Input: part model. Units: mm. Frame: model coordinates. A direction names the side the tool comes from. Round coordinates to 2 decimals unless told otherwise and drop trailing zeros. Write each loop counter-clockwise with the first axis right and the second up, starting at its lowest first coordinate (ties: lowest second). Pieces come first, ordered by that corner, then holes. Notation, with made-up numbers: (34.25, 76) - (83.25, 76) arc R29 ccw to (83.25, 109) - close; hole circle Ø4 at (27.25, 52). An arc over 180 degrees is marked (long way). Use one line per item in the form item = value.
```python
from build123d import *

# Parameters (mm, degrees)
SKETCH1_W                      = 38.1
SKETCH1_H                      = 50.8
SKETCH1_W_2                    = 31.75
SKETCH1_H_2                    = 44.45
BOSS_EXTRUDE1_DEPTH            = 152.4
SKETCH2_R                      = 1.89865
CUT_EXTRUDE1_DEPTH             = 35.925
CUT_EXTRUDE1_DEPTH_BACK        = 4.175
CUT_EXTRUDE3_DEPTH             = 3.175
CUT_EXTRUDE4_DEPTH             = 3.175
SKETCH6_R                      = 9.525
SKETCH6_R_2                    = 2.5527
CUT_EXTRUDE5_DEPTH             = 3.175
CUT_EXTRUDE6_DEPTH             = 3.175
F_6_32_TAPPED_HOLE2_D          = 2.7051
F_6_32_TAPPED_HOLE2_DEPTH      = 3.175
CUT_EXTRUDE7_REACH             = 40.1
CUT_EXTRUDE7_DIRECTION_2_DEPTH = 1
FILLET1_R                      = 3.175
FILLET2_R                      = 3.175
BOSS_EXTRUDE2_DEPTH            = 3.175
CUT_EXTRUDE8_REACH             = 40.1
FILLET3_R                      = 3.175
FILLET4_R                      = 3.175
FILLET5_R                      = 6.35
FILLET6_R                      = 6.35
BOSS_EXTRUDE3_DEPTH            = 3.175
CUT_EXTRUDE9_REACH             = 40.1
BOSS_EXTRUDE4_DEPTH            = 3.175
FILLET7_R                      = 3.175
FILLET8_R                      = 3.175
FILLET9_R                      = 3.175
FILLET10_R                     = 3.175
FILLET11_R                     = 6.35
FILLET12_R                     = 6.35


with BuildPart() as part:
    # Sketch1 → Boss-Extrude1 (new body)
    with BuildSketch(Plane(origin=(0, 0, 0), x_dir=(1, 0, 0), z_dir=(0, 1, 0))):
        Rectangle(SKETCH1_W, SKETCH1_H)
        Rectangle(SKETCH1_W_2, SKETCH1_H_2, mode=Mode.SUBTRACT)
    extrude(amount=BOSS_EXTRUDE1_DEPTH)

    # Sketch2 → Cut-Extrude1 (cut, two sides)
    with BuildSketch(Plane.ZY.offset(-15.875)) as cut_extrude1_sk:
        with Locations((-16.645384182, 6.21538)):
            Circle(SKETCH2_R)
        with Locations((10.30030417, 6.18241423)):
            Circle(SKETCH2_R)
    extrude(amount=CUT_EXTRUDE1_DEPTH, mode=Mode.SUBTRACT)
    extrude(cut_extrude1_sk.sketch, amount=-CUT_EXTRUDE1_DEPTH_BACK, mode=Mode.SUBTRACT)

    # Sketch4 → Cut-Extrude3 (cut)
    with BuildSketch(Plane.ZY.offset(19.05)):
        with BuildLine():
            Line((17.4625, 10.16), (-17.4625, 10.16))
            ThreePointArc((-17.4625, 10.16), (-19.70756403, 11.08993597), (-20.6375, 13.335))
            Line((-20.6375, 13.335), (-20.6375, 64.135))
            ThreePointArc((-20.6375, 64.135), (-19.70756403, 66.38006403), (-17.4625, 67.31))
            Line((-17.4625, 67.31), (17.4625, 67.31))
            ThreePointArc((17.4625, 67.31), (19.70756403, 66.38006403), (20.6375, 64.135))
            Line((20.6375, 64.135), (20.6375, 13.335))
            ThreePointArc((20.6375, 13.335), (19.70756403, 11.08993597), (17.4625, 10.16))
        make_face()
    extrude(amount=-CUT_EXTRUDE3_DEPTH, mode=Mode.SUBTRACT)

    # Sketch5 → Cut-Extrude4 (cut)
    with BuildSketch(Plane(origin=(19.05, 0, 0), x_dir=(0, 0, -1), z_dir=(1, 0, 0))):
        with BuildLine():
            Line((17.4625, 67.31), (-17.4625, 67.31))
            ThreePointArc((-17.4625, 67.31), (-19.70756403, 66.38006403), (-20.6375, 64.135))
            Line((-20.6375, 64.135), (-20.6375, 45.085))
            ThreePointArc((-20.6375, 45.085), (-19.70756403, 42.83993597), (-17.4625, 41.91))
            Line((-17.4625, 41.91), (17.4625, 41.91))
            ThreePointArc((17.4625, 41.91), (19.70756403, 42.83993597), (20.6375, 45.085))
            Line((20.6375, 45.085), (20.6375, 64.135))
            ThreePointArc((20.6375, 64.135), (19.70756403, 66.38006403), (17.4625, 67.31))
        make_face()
    extrude(amount=-CUT_EXTRUDE4_DEPTH, mode=Mode.SUBTRACT)

    # Sketch6 → Cut-Extrude5 (cut)
    with BuildSketch(Plane.ZY.offset(-15.875)):
        with Locations((0, 101.6)):
            Circle(SKETCH6_R)
        with Locations((0, 87.63)):
            Circle(SKETCH6_R_2)
        with Locations((-9.878281733, 91.721718267)):
            Circle(SKETCH6_R_2)
        with Locations((-13.97, 101.6)):
            Circle(SKETCH6_R_2)
        with Locations((-9.878281733, 111.478281733)):
            Circle(SKETCH6_R_2)
        with Locations((0, 115.57)):
            Circle(SKETCH6_R_2)
        with Locations((9.878281733, 111.478281733)):
            Circle(SKETCH6_R_2)
        with Locations((13.97, 101.6)):
            Circle(SKETCH6_R_2)
        with Locations((9.878281733, 91.721718267)):
            Circle(SKETCH6_R_2)
    extrude(amount=-CUT_EXTRUDE5_DEPTH, mode=Mode.SUBTRACT)

    # Sketch7 → Cut-Extrude6 (cut)
    with BuildSketch(Plane.ZY.offset(19.05)):
        with BuildLine():
            Line((-14.2875, 77.47), (14.2875, 77.47))
            ThreePointArc((14.2875, 77.47), (18.777628061, 79.329871939), (20.6375, 83.82))
            Line((20.6375, 83.82), (20.6375, 121.92))
            ThreePointArc((20.6375, 121.92), (18.777628061, 126.410128061), (14.2875, 128.27))
            Line((14.2875, 128.27), (-14.2875, 128.27))
            ThreePointArc((-14.2875, 128.27), (-18.777628061, 126.410128061), (-20.6375, 121.92))
            Line((-20.6375, 121.92), (-20.6375, 83.82))
            ThreePointArc((-20.6375, 83.82), (-18.777628061, 79.329871939), (-14.2875, 77.47))
        make_face()
    extrude(amount=-CUT_EXTRUDE6_DEPTH, mode=Mode.SUBTRACT)

    # #6-32 Tapped Hole2
    with Locations(Plane(origin=(5.579615818, 136.6393, -25.4), x_dir=(-1, 0, 0), z_dir=(0, 0, -1))):
        with Locations((0, 0), (11.159231636, 0)):
            Hole(F_6_32_TAPPED_HOLE2_D / 2, depth=F_6_32_TAPPED_HOLE2_DEPTH)

    # Sketch13 → Cut-Extrude7 (cut, up to next)
    with BuildSketch(Plane(origin=(19.05, 0, 0), x_dir=(0, 0, -1), z_dir=(1, 0, 0)), mode=Mode.PRIVATE) as cut_extrude7_sk1:
        Polygon((0, 78.486), (20.6375, 78.486), (20.6375, 64.135), (-20.6375, 64.135), (-20.6375, 78.486), align=None)
    cut_extrude7_tool1 = extrude(cut_extrude7_sk1.sketch, amount=-CUT_EXTRUDE7_REACH, mode=Mode.PRIVATE) & part.part
    add(cut_extrude7_tool1.solids().sort_by_distance((19.05, 71.3105, 0))[0], mode=Mode.SUBTRACT)

    # Sketch13 → Cut-Extrude7 direction 2 (cut)
    with BuildSketch(Plane(origin=(19.05, 0, 0), x_dir=(0, 0, -1), z_dir=(1, 0, 0))):
        Polygon((0, 78.486), (20.6375, 78.486), (20.6375, 64.135), (-20.6375, 64.135), (-20.6375, 78.486), align=None)
    extrude(amount=CUT_EXTRUDE7_DIRECTION_2_DEPTH, mode=Mode.SUBTRACT)

    # Fillet1
    fillet1_edges = [part.edges().sort_by_distance(p)[0] for p in [
        (17.4625, 78.486, -20.6375),
    ]]
    fillet(fillet1_edges, radius=FILLET1_R)

    # Fillet2
    fillet2_edges = [part.edges().sort_by_distance(p)[0] for p in [
        (17.4625, 78.486, 20.6375),
    ]]
    fillet(fillet2_edges, radius=FILLET2_R)

    # Sketch15 → Boss-Extrude2 (add)
    with BuildSketch(Plane.ZY.offset(19.05)):
        Polygon((0, 78.486), (-20.6375, 78.486), (-20.6375, 88.646), (0, 88.646), (20.6375, 88.646), (20.6375, 78.486), align=None)
    extrude(amount=-BOSS_EXTRUDE2_DEPTH)

    # Sketch16 → Cut-Extrude8 (cut, up to next)
    with BuildSketch(Plane.ZY.offset(19.05), mode=Mode.PRIVATE) as cut_extrude8_sk1:
        Polygon((0, 78.486), (20.6375, 78.486), (20.6375, 64.135), (-20.6375, 64.135), (-20.6375, 78.486), align=None)
    cut_extrude8_tool1 = extrude(cut_extrude8_sk1.sketch, amount=-CUT_EXTRUDE8_REACH, mode=Mode.PRIVATE) & part.part
    add(cut_extrude8_tool1.solids().sort_by_distance((-19.05, 71.3105, 0))[0], mode=Mode.SUBTRACT)

    # Fillet3
    fillet3_edges = [part.edges().sort_by_distance(p)[0] for p in [
        (-17.4625, 78.486, 20.6375),
    ]]
    fillet(fillet3_edges, radius=FILLET3_R)

    # Fillet4
    fillet4_edges = [part.edges().sort_by_distance(p)[0] for p in [
        (-17.4625, 78.486, -20.6375),
    ]]
    fillet(fillet4_edges, radius=FILLET4_R)

    # Fillet5
    fillet5_edges = [part.edges().sort_by_distance(p)[0] for p in [
        (-17.4625, 88.646, -20.6375),
    ]]
    fillet(fillet5_edges, radius=FILLET5_R)

    # Fillet6
    fillet6_edges = [part.edges().sort_by_distance(p)[0] for p in [
        (-17.4625, 88.646, 20.6375),
    ]]
    fillet(fillet6_edges, radius=FILLET6_R)

    # Sketch17 → Boss-Extrude3 (add)
    with BuildSketch(Plane.ZY.offset(19.05)):
        Polygon((0, 74.168), (20.6375, 74.168), (20.6375, 84.35471455), (-20.6375, 84.35471455), (-20.6375, 74.168), align=None)
    extrude(amount=-BOSS_EXTRUDE3_DEPTH)

    # Sketch18 → Cut-Extrude9 (cut, up to next)
    with BuildSketch(Plane.ZY.offset(19.05), mode=Mode.PRIVATE) as cut_extrude9_sk1:
        Polygon((0, 84.328), (-20.6375, 84.328), (-20.6375, 94.996), (20.6375, 94.996), (20.6375, 84.328), align=None)
    cut_extrude9_tool1 = extrude(cut_extrude9_sk1.sketch, amount=-CUT_EXTRUDE9_REACH, mode=Mode.PRIVATE) & part.part
    add(cut_extrude9_tool1.solids().sort_by_distance((-19.05, 89.662, 0))[0], mode=Mode.SUBTRACT)

    # Sketch19 → Boss-Extrude4 (add)
    with BuildSketch(Plane(origin=(19.05, 0, 0), x_dir=(0, 0, -1), z_dir=(1, 0, 0))):
        Polygon((0, 74.168), (20.6375, 74.168), (20.6375, 78.486), (-20.6375, 78.486), (-20.6375, 74.168), align=None)
    extrude(amount=-BOSS_EXTRUDE4_DEPTH)

    # Fillet7
    fillet7_edges = [part.edges().sort_by_distance(p)[0] for p in [
        (17.4625, 74.168, -20.6375),
    ]]
    fillet(fillet7_edges, radius=FILLET7_R)

    # Fillet8
    fillet8_edges = [part.edges().sort_by_distance(p)[0] for p in [
        (17.4625, 74.168, 20.6375),
    ]]
    fillet(fillet8_edges, radius=FILLET8_R)

    # Fillet9
    fillet9_edges = [part.edges().sort_by_distance(p)[0] for p in [
        (-17.4625, 74.168, 20.6375),
    ]]
    fillet(fillet9_edges, radius=FILLET9_R)

    # Fillet10
    fillet10_edges = [part.edges().sort_by_distance(p)[0] for p in [
        (-17.4625, 74.168, -20.6375),
    ]]
    fillet(fillet10_edges, radius=FILLET10_R)

    # Fillet11
    fillet11_edges = [part.edges().sort_by_distance(p)[0] for p in [
        (-17.4625, 84.328, -20.6375),
    ]]
    fillet(fillet11_edges, radius=FILLET11_R)

    # Fillet12
    fillet12_edges = [part.edges().sort_by_distance(p)[0] for p in [
        (-17.4625, 84.328, 20.6375),
    ]]
    fillet(fillet12_edges, radius=FILLET12_R)


solid = part.part
```
(1) Cut plane A-A on y = 101.6. Count the separate pieces of the cut face and the enclosed holes in it, then the cut area to 3 significant figures.
Derived:
separate_pieces = 4
enclosed_holes = 0
area = 300 mm^2
(2) Access query for faces 4 (the face through (-17, 42, -20.638)), 5 (the face through (0, 75, 22.225)), 6 (the face through (17, 74.168, 0)). Directions: +Z, -Z, +X, -X, +Y, -Y. A direction counts if a zero-diameter tool reaches every point of the face in a straight line with its end or side. Return the directions, or none.
Derived:
face_4 = -X
face_5 = +Y, -Y
face_6 = +X, -X
(3) Cut plane C-C on z = 19. Output: boundary loops of the cut face in (x, y) (3 decimals).
Derived:
outline = (-19.05, 0) - (-15.875, 0) - (-15.875, 10.557) - (-19.05, 10.557) - close; (-19.05, 73.771) - (-15.875, 73.771) - (-15.875, 86.422) - (-19.05, 86.422) - close; (-19.05, 126.176) - (-15.875, 126.176) - (-15.875, 152.4) - (-19.05, 152.4) - close; (15.875, 0) - (19.05, 0) - (19.05, 42.307) - (15.875, 42.307) - close; (15.875, 73.771) - (19.05, 73.771) - (19.05, 152.4) - (15.875, 152.4) - close
(4) Material intervals for L1, parallel to Y at x = 17.65, z = 0 (3 decimals); L2, parallel to Y at x = -16.5, z = -11; L3, parallel to X at y = 128, z = -22 (3 decimals), sorted ascending.
Derived:
L1 = 0 to 41.91, 74.168 to 85.077, 90.183 to 92.075, 111.125 to 113.017, 118.123 to 152.4
L2 = 0 to 10.16, 74.17 to 84.33, 128.27 to 152.4
L3 = -19.05 to -15.875, 15.875 to 19.05
(5) First-contact query: pin 1 Ø3 at (y, z) = (108.5, -11) entering from -X (3 decimals); pin 2 Ø25 at (y, z) = (101.6, 0) entering from +X. Flat tips, straight axial feed; report the tip coordinate or a pass-through.
Derived:
pin_1 = 15.875
pin_2 = 19.05
(6) Cut plane B-B on x = 14.5. Output: boundary loops of the cut face in (y, z) (3 decimals).
Derived:
outline = (0, -25.4) - (152.4, -25.4) - (152.4, -22.225) - (0, -22.225) - close; (0, 22.225) - (152.4, 22.225) - (152.4, 25.4) - (0, 25.4) - close
(7) Draft query along Z for faces 1 (the face through (0, 75, -25.4)), 2 (the face through (-19.05, 77, 0)), 3 (the face through (-17.44, 4.362, -17.057)). Return one class per face: released by +Z, released by -Z, zero draft, split by the parting line, or undercut.
Derived:
face_1 = released by -Z
face_2 = zero draft
face_3 = undercut
